CAD build for the part. Positions are in the model's coordinates, mm. Coordinates: 2 decimals unless noted, no trailing zeros. Order: outer loops, then holes, each group sorted by start corner. A loop starts at its lowest first (then second) coordinate and runs counter-clockwise, first axis right, second up. Notation, with made-up numbers: (1, 40) - (49, 40) arc R12 ccw to (49, 60) - close; hole circle Ø6 at (-34.5, -26). An arc over 180 degrees is marked (long way). Return JSON: item names as keys, results as strings.
Autodesk Inventor part; units mm, degrees
ref_plane "YZ Plane" through (0, 0, 0) normal (1, 0, 0) x (0, 1, 0)
ref_plane "XZ Plane" through (0, 0, 0) normal (0, 1, 0) x (-1, 0, 0)
ref_plane "XY Plane" through (0, 0, 0) normal (0, 0, 1) x (1, 0, 0)
sketch "Sketch1" plane through (0, 0, 0) normal (0, 0, 1) x (1, 0, 0)
  line L0 (7.62, 0) -> (12.065, 0)
  line L1 (15.24, 3.175) -> (15.24, 47.625)
  line L2 (12.065, 50.8) -> (7.62, 50.8)
  circle A0 centre (7.62, 44.45) radius 4.1656
  circle A1 centre (7.62, 6.35) radius 4.1656
  arc A2 (15.24, 47.625) -> (12.065, 50.8) centre (12.065, 47.625) ccw
  arc A3 (12.065, 0) -> (15.24, 3.175) centre (12.065, 3.175) ccw
  circle A4 centre (-69.85, 25.4) radius 3.175
  arc A5 (-71.3663, 31.5663) -> (-71.3663, 19.2337) centre (-69.85, 25.4) ccw
  arc A6 (7.62, 50.8) -> (6.1037, 50.6163) centre (7.62, 44.45) ccw
  arc A7 (6.1037, 0.1837) -> (7.62, 0) centre (7.62, 6.35) ccw
  line L3 (-69.85, 25.4) -> (7.62, 44.45) construction
  line L4 (-69.85, 25.4) -> (7.62, 6.35) construction
  line L5 (15.24, 25.4) -> (-69.85, 25.4) construction
  line L6 (-71.3663, 31.5663) -> (6.1037, 50.6163)
  line L7 (-71.3663, 19.2337) -> (6.1037, 0.1837)
  line L8 (0, 42.5762) -> (0, 0) construction
  point P0 (15.24, 50.8)
  point P1 (15.24, 0)
  dimension "d1" = 50.8
  dimension "d2" = 38.1
  dimension "d3" = 6.35
  dimension "d4" = 8.3312
  dimension "d5" = 8.3312
  dimension "d9" = 3.175
  dimension "d12" = 6.35
  dimension "d14" = 12.7
  dimension "d16" = 15.24
  dimension "d18" = 76.185
  dimension "d19" = 50.8
  dimension "d20" = 25.4
  dimension "d21" = 85.09
  dimension "d22" = 69.85
  dimension "d23" = 76.185
  dimension "d24" = 27.63
  dimension "d25" = 27.63
  dimension "d26" = 152.37
  dimension "d27" = 13.815
  dimension "d28" = 4.445
  dimension "d29" = 77.47
  dimension "d30" = 19.05
  dimension "d31" = 13.815
  dimension "d32" = 13.815
  dimension "d33" = 7.62
  dimension "d34" = 6.35
  dimension "d35" = 90
  dimension "d36" = 7.62
  dimension "d37" = 6.35
  dimension "d38" = 4.445
  dimension "d39" = 3.175
extrude "Extrusion1" add sketch "Sketch1" along normal blind 3.175
equation "\"d5\" = d4"
properties part number "pully mount"
Item 1: Band-saw the part on C-C, the plane x = -69. List the corners of the cut face in (y, z) (3 decimals).
Findings below:
{"outline": "(18.652, 0) - (22.341, 0) - (22.341, 3.175) - (18.652, 3.175) - close; (28.459, 0) - (32.148, 0) - (32.148, 3.175) - (28.459, 3.175) - close"}
Item 2: Band-saw the part on D-D, the plane x = -26.5. List the corners of the cut face in (y, z) (3 decimals), then the cut area to 3 significant figures.
Findings below:
{"outline": "(8.201, 0) - (42.599, 0) - (42.599, 3.175) - (8.201, 3.175) - close", "area": "109 mm²"}
Item 3: Band-saw the part on A-A, the plane z = 2.1. List the corners of the cut face in (x, y) (3 decimals), then the cut area to 3 significant figures.
Findings below:
{"outline": "(-71.366, 19.234) - (6.104, 0.184) arc R6.35 ccw to (7.62, 0) - (12.065, 0) arc R3.175 ccw to (15.24, 3.175) - (15.24, 47.625) arc R3.175 ccw to (12.065, 50.8) - (7.62, 50.8) arc R6.35 ccw to (6.104, 50.616) - (-71.366, 31.566) arc R6.35 ccw to start; hole circle Ø6.35 at (-69.85, 25.4); hole circle Ø8.331 at (7.62, 6.35); hole circle Ø8.331 at (7.62, 44.45)", "area": "2,790 mm²"}
Item 4: Drop flat-ended pins along their axis: P1, Ø4, axis at x = -69.85, y = 25.4, coming from the -Z side; P2, Ø1.5, axis at x = -39.5, z = 2.5, coming from the -Y side; P3, Ø5, axis at x = -27, y = 43, coming from the +Z side (3 decimals). Give the stop position or say it passes through.
Findings below:
{"P1": "passes through", "P2": "stops at y = 11.21", "P3": "stops at z = 3.175"}
Item 5: Wall check: L1, parallel to Y at x = 7.62, z = 1.8; L2, parallel to X at y = 25.5, z = 1.35; L3, parallel to Y at x = -6, z = 0.2. Give the ranges that are in metal, low to high. Write a range as [from, to].
Findings below:
{"L1": "y = [0, 2.18], [10.52, 40.28], [48.62, 50.8]", "L2": "x = [-76.2, -73.02], [-66.68, 15.24]", "L3": "y = [3.16, 47.64]"}
Item 6: Band-saw the part on B-B, the plane y = 25.4. List the corners of the cut face in (x, z) (3 decimals).
Findings below:
{"outline": "(-76.2, 0) - (-73.025, 0) - (-73.025, 3.175) - (-76.2, 3.175) - close; (-66.675, 0) - (15.24, 0) - (15.24, 3.175) - (-66.675, 3.175) - close"}
Item 7: Mould opens along X. For faces 1 (the cylindrical face through (3.46, 6.17, 1.57)), 2 (the cylindrical face through (14.29, 49.89, 1.57)), 3 (the cylindrical face through (6.717, 48.517, 1.565)), 4 (the cylindrical face through (-76.2, 25.3, 1.6)) say: released by +X, released by -X, zero draft, split by the parting line, or undercut.
Findings below:
{"face 1": "undercut", "face 2": "released by +X", "face 3": "undercut", "face 4": "released by -X"}
